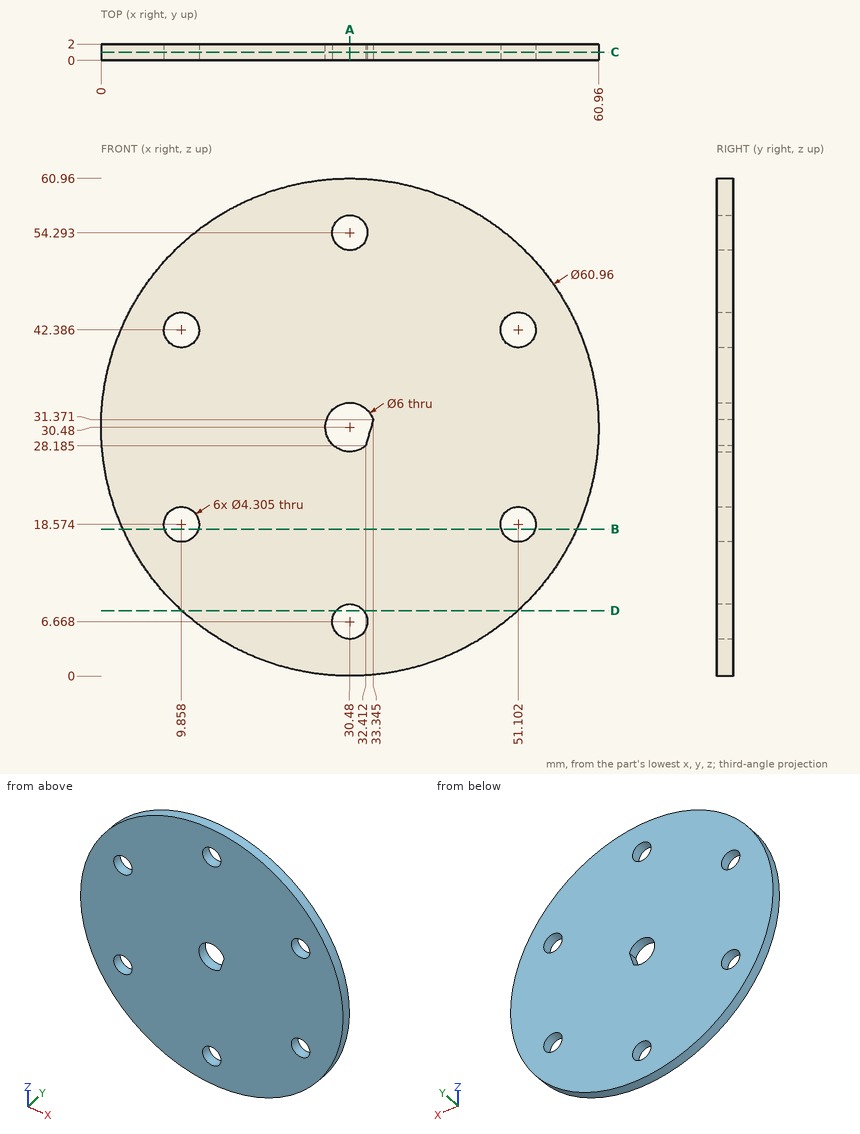
The drawing under review shows one solid part. Ordinate dimensions are in mm from its lowest x, y, z. Round coordinates to 2 decimals unless told otherwise and drop trailing zeros. Write each loop counter-clockwise with the first axis right and the second up, starting at its lowest first coordinate (ties: lowest second). Pieces come first, ordered by that corner, then holes. Notation, with made-up numbers: (-25, -18) -> (29, -18) arc R17 ccw to (29, 5) -> close; hole circle Ø7 at (45, 84.5). An arc over 180 degrees is marked (long way). Put each result on its own line as item: value.
Q1. To check wall thickness, follow L1, parallel to Z at x = 52, y = 0.85 (1 decimal); L2, parallel to Z at x = 29, y = 1.1 (1 decimal); L3, parallel to X at y = 1.8, z = 53. State the ranges of each line that lie inside material, in increasing order. Write a range as [from, to].
Determined:
L1: z = [8.9, 16.6], [20.5, 40.4], [44.3, 52.1]
L2: z = [0, 5.1], [8.2, 27.9], [33.1, 52.7], [55.9, 60.9]
L3: x = [9.94, 28.76], [32.2, 51.02]
Q2. Consider section A-A on x = 30.48. State the section outline as (y, z) points (1 decimal).
Determined:
outline: (0, 0) -> (2, 0) -> (2, 4.5) -> (0, 4.5) -> close; (0, 8.8) -> (2, 8.8) -> (2, 27.5) -> (0, 27.5) -> close; (0, 33.5) -> (2, 33.5) -> (2, 52.1) -> (0, 52.1) -> close; (0, 56.4) -> (2, 56.4) -> (2, 61) -> (0, 61) -> close
Q3. Consider section C-C on y = 1. State the section outline as (x, z) points (1 decimal).
Determined:
outline: circle Ø61 at (30.5, 30.5); hole circle Ø4.3 at (9.9, 18.6); hole circle Ø4.3 at (9.9, 42.4); hole circle Ø4.3 at (30.5, 6.7); hole circle Ø4.3 at (30.5, 54.3); hole (32.4, 28.2) -> (33.3, 31.4) arc R3 ccw (long way) to start; hole circle Ø4.3 at (51.1, 18.6); hole circle Ø4.3 at (51.1, 42.4)
Q4. Consider section B-B on z = 18. State the section outline as (x, y) points.
Determined:
outline: (2.67, 0) -> (7.78, 0) -> (7.78, 2) -> (2.67, 2) -> close; (11.93, 0) -> (49.03, 0) -> (49.03, 2) -> (11.93, 2) -> close; (53.18, 0) -> (58.29, 0) -> (58.29, 2) -> (53.18, 2) -> close
Q5. Clearance check with a flat-ended pin moving along its axis: pin 1 Ø9.5 at (x, z) = (30.48, 30.48) entering from +Y. State where the tip first meets the part, or that it passes through.
Determined:
pin 1: stops at y = 2
Q6. Consider section D-D on z = 8. State the section outline as (x, y) points.
Determined:
outline: (9.9, 0) -> (28.79, 0) -> (28.79, 2) -> (9.9, 2) -> close; (32.17, 0) -> (51.06, 0) -> (51.06, 2) -> (32.17, 2) -> close
